```python
from build123d import *

# Parameters (mm, degrees)
SKETCH1_W             = 91
SKETCH1_H             = 38
SKETCH1_R             = 3
BOSS_EXTRUDE1_DEPTH   = 10
M3X0_5_TAPPED_HOLE1_D = 2.5


with BuildPart() as part:
    # Sketch1 → Boss-Extrude1 (new body)
    with BuildSketch(Plane(origin=(0, 0, 0), x_dir=(1, 0, 0), z_dir=(0, 1, 0))):
        with Locations((26.530497816, -16.359463259)):
            Rectangle(SKETCH1_W, SKETCH1_H)
        with Locations(Location((41.030497816, -28.859463259, 0), (0, 0, 270))):
            Circle(SKETCH1_R, mode=Mode.SUBTRACT)
        with Locations(Location((66.030497816, -28.859463259, 0), (0, 0, 270))):
            Circle(SKETCH1_R, mode=Mode.SUBTRACT)
        with Locations(Location((41.030497816, -3.859463259, 0), (0, 0, 270))):
            Circle(SKETCH1_R, mode=Mode.SUBTRACT)
        with Locations(Location((66.030497816, -3.859463259, 0), (0, 0, 270))):
            Circle(SKETCH1_R, mode=Mode.SUBTRACT)
    extrude(amount=BOSS_EXTRUDE1_DEPTH)

    # M3x0.5 Tapped Hole1 (through all)
    with Locations(Plane(origin=(0, 0, 0), x_dir=(-1, 0, 0), z_dir=(0, -1, 0))):
        with Locations((-16.030497816, -0.359463259), (15.969502184, -32.359463259), (-16.030497816, -32.359463259), (15.969502184, -0.359463259)):
            Hole(M3X0_5_TAPPED_HOLE1_D / 2)


solid = part.part
```
Input: part model. Units: mm. Frame: model coordinates. Coordinates: 2 decimals unless noted, no trailing zeros. Use one line per item in the form item = value.
Q1. Material intervals for probe 1 along Z at (x, y) = (66, 8.5); probe 2 along X at (y, z) = (0.5, 6.5); probe 3 along X at (y, z) = (6, 26.5), sorted ascending. Write a range as from..to.
Answer below:
probe_1 = -2.64..0.86, 6.86..25.86, 31.86..35.36
probe_2 = -18.97..39.61, 42.45..64.61, 67.45..72.03
probe_3 = -18.97..39.18, 42.88..64.18, 67.88..72.03
Q2. Draft query along X for faces 1 (the face through (26, 0, 16)), 2 (the face through (38.1, 4.93, 3.21)), 3 (the face through (-18.97, 5, 17)). Return one class per face: released by +X, released by -X, zero draft, split by the parting line, or undercut.
Answer below:
face_1 = zero draft
face_2 = undercut
face_3 = released by -X
Q3. First-contact query: pin 1 (12 mm diameter, centred on x = 15.5, z = 7.5, fed in from -Y). Flat tip, straight axial feed; report the tip coordinate or a pass-through.
Answer below:
pin_1 = 0
Q4. Section A-A (y = 5). Count the separate pieces of the cut face and the enclosed holes in it, plus the area to 3 significant figures.
Answer below:
separate_pieces = 1
enclosed_holes = 8
area = 3,330 mm²
